Verification items for the finished model (mm, model axes). Coordinates: 2 decimals unless noted, no trailing zeros. Write each loop counter-clockwise with the first axis right and the second up, starting at its lowest first coordinate (ties: lowest second). Pieces come first, ordered by that corner, then holes. Notation, with made-up numbers: (63.5, 39) -> (98.5, 39) arc R22 cw to (98.5, 56) -> close; hole circle Ø7 at (-31.5, 73). An arc over 180 degrees is marked (long way). Answer in a Markdown table with one row per item.
```python
from build123d import *

# Parameters (mm, degrees)
SKETCH1_R                           = 23
BOSS_EXTRUDE1_DEPTH                 = 75
CUT_EXTRUDE1_REACH                  = 83.75
CUT_EXTRUDE1_END_RADIUS             = 23
SKETCH2_R                           = 13.709861361
SKETCH2_R_2                         = 12.670153282
CUT_EXTRUDE1_DIRECTION_2_REACH      = 83.75
CUT_EXTRUDE1_DIRECTION_2_END_RADIUS = 23


with BuildPart() as part:
    # Sketch1 → Boss-Extrude1 (new body)
    with BuildSketch(Plane(origin=(0, 0, 0), x_dir=(0, 0, -1), z_dir=(1, 0, 0))):
        Circle(SKETCH1_R)
    extrude(amount=BOSS_EXTRUDE1_DEPTH)

    # Cut-Extrude1: up to this cylinder (the profile starts inside it)
    cut_extrude1_end = Plane(origin=(37.49105, 0, 0), z_dir=(-1, 0, 0)) * Cylinder(CUT_EXTRUDE1_END_RADIUS, 289.4821, mode=Mode.PRIVATE)
    # Sketch2 → Cut-Extrude1 (cut, up to the surface)
    with BuildSketch(Plane.XY, mode=Mode.PRIVATE) as cut_extrude1_sk1:
        Circle(SKETCH2_R)
    cut_extrude1_tool1 = extrude(cut_extrude1_sk1.sketch, amount=-CUT_EXTRUDE1_REACH, mode=Mode.PRIVATE) & cut_extrude1_end
    add(cut_extrude1_tool1.solids().sort_by_distance((0, 0, 0))[0], mode=Mode.SUBTRACT)
    # Sketch2 → Cut-Extrude1 (cut, up to the surface)
    with BuildSketch(Plane.XY, mode=Mode.PRIVATE) as cut_extrude1_sk2:
        with Locations((74.982099517, 0)):
            Circle(SKETCH2_R_2)
    cut_extrude1_tool2 = extrude(cut_extrude1_sk2.sketch, amount=-CUT_EXTRUDE1_REACH, mode=Mode.PRIVATE) & cut_extrude1_end
    add(cut_extrude1_tool2.solids().sort_by_distance((74.9821, 0, 0))[0], mode=Mode.SUBTRACT)

    # Cut-Extrude1 direction 2: up to this cylinder (the profile starts inside it)
    cut_extrude1_direction_2_end = Plane(origin=(37.49105, 0, 0), z_dir=(-1, 0, 0)) * Cylinder(CUT_EXTRUDE1_DIRECTION_2_END_RADIUS, 289.4821, mode=Mode.PRIVATE)
    # Sketch2 → Cut-Extrude1 direction 2 (cut, up to the surface)
    with BuildSketch(Plane.XY, mode=Mode.PRIVATE) as cut_extrude1_direction_2_sk1:
        Circle(SKETCH2_R)
    cut_extrude1_direction_2_tool1 = extrude(cut_extrude1_direction_2_sk1.sketch, amount=CUT_EXTRUDE1_DIRECTION_2_REACH, mode=Mode.PRIVATE) & cut_extrude1_direction_2_end
    add(cut_extrude1_direction_2_tool1.solids().sort_by_distance((0, 0, 0))[0], mode=Mode.SUBTRACT)
    # Sketch2 → Cut-Extrude1 direction 2 (cut, up to the surface)
    with BuildSketch(Plane.XY, mode=Mode.PRIVATE) as cut_extrude1_direction_2_sk2:
        with Locations((74.982099517, 0)):
            Circle(SKETCH2_R_2)
    cut_extrude1_direction_2_tool2 = extrude(cut_extrude1_direction_2_sk2.sketch, amount=CUT_EXTRUDE1_DIRECTION_2_REACH, mode=Mode.PRIVATE) & cut_extrude1_direction_2_end
    add(cut_extrude1_direction_2_tool2.solids().sort_by_distance((74.9821, 0, 0))[0], mode=Mode.SUBTRACT)


solid = part.part
```
1. Sectioned sample at D-D, the plane y = -19. Record the cut outline in (x, z).
Findings below:
| item | result |
|---|---|
| outline | (0, -12.96) -> (75, -12.96) -> (75, 12.96) -> (0, 12.96) -> close |
2. Material ranges on probe 1 along Y at (x, z) = (65, -6.5); probe 2 along Z at (x, y) = (70.5, -16); probe 3 along Y at (x, z) = (38, -14.5), recorded low to high. Write a range as from..to.
Findings below:
| item | result |
|---|---|
| probe 1 | y = -22.06..-7.8, 7.8..22.06 |
| probe 2 | z = -16.52..16.52 |
| probe 3 | y = -17.85..17.85 |
3. Go/stop test with flat-tipped pins: pin 1 (3 mm diameter, centred on x = 47.5, z = 3.5, fed in from +Y); pin 2 (3 mm diameter, centred on x = 10, z = 7.5, fed in from -Y); pin 3 (2 mm diameter, centred on x = 19, z = 9.5, fed in from -Y). Record where each tip stops, or that it passes through.
Findings below:
| item | result |
|---|---|
| pin 1 | stops at y = 22.91 |
| pin 2 | stops at y = -22.2 |
| pin 3 | stops at y = -21.37 |
4. Sectioned sample at C-C, the plane x = 29. Record the cut outline in (y, z).
Findings below:
| item | result |
|---|---|
| outline | circle Ø46 at (0, 0) |
5. Release check for a two-part mould opening along Y. For faces 1 (the face through (36.975, 1.011, 22.978)), 2 (the face through (13.707, -0.301, 0.323)), 3 (the face through (0, 17, 0)) record: released by +Y, released by -Y, zero draft, split by the parting line, or undercut.
Findings below:
| item | result |
|---|---|
| face 1 | split by the parting line |
| face 2 | undercut |
| face 3 | zero draft |
6. Sectioned sample at A-A, the plane z = 0. Record the cut outline in (x, y), and give its area (3 significant figures).
Findings below:
| item | result |
|---|---|
| outline | (0, -23) -> (75, -23) -> (75, -12.67) arc R12.67 cw to (75, 12.67) -> (75, 23) -> (0, 23) -> (0, 13.71) arc R13.71 cw to (0, -13.71) -> close |
| area | 2,900 mm² |
7. Sectioned sample at B-B, the plane x = 67. Record the cut outline in (y, z), and give its area (3 significant figures).
Findings below:
| item | result |
|---|---|
| outline | (-9.84, -20.79) -> (-9.84, 20.79) arc R23 ccw to start; (9.84, -20.79) arc R23 ccw to (9.84, 20.79) -> close |
| area | 785 mm² |
